from build123d import *

# Parameters (mm, degrees)
SKETCH_1_W      = 42
SKETCH_1_H      = 60
SKETCH_1_R      = 8
SKETCH_1_R_2    = 1.6
SKETCH_1_R_3    = 2.5
EXTRUDE_1_DEPTH = 2


with BuildPart() as part:
    # 草图1 → 凸台-拉伸1 (new body)
    with BuildSketch(Plane.XY):
        with Locations((0, -9)):
            Rectangle(SKETCH_1_W, SKETCH_1_H)
        Circle(SKETCH_1_R, mode=Mode.SUBTRACT)
        with Locations((-15.5, 15.5)):
            Circle(SKETCH_1_R_2, mode=Mode.SUBTRACT)
        with Locations((-15.5, -15.5)):
            Circle(SKETCH_1_R_2, mode=Mode.SUBTRACT)
        with Locations((-12.5, -31)):
            Circle(SKETCH_1_R_3, mode=Mode.SUBTRACT)
        with Locations(Location((15.5, 15.5, 0), (0, 0, 180))):
            Circle(SKETCH_1_R_2, mode=Mode.SUBTRACT)
        with Locations(Location((15.5, -15.5, 0), (0, 0, 180))):
            Circle(SKETCH_1_R_2, mode=Mode.SUBTRACT)
        with Locations(Location((12.5, -31, 0), (0, 0, 180))):
            Circle(SKETCH_1_R_3, mode=Mode.SUBTRACT)
    extrude(amount=EXTRUDE_1_DEPTH)


solid = part.part
Source: CAD feature listing. Evaluate the final solid. Frame: model axes, mm. Round coordinates to 2 decimals unless told otherwise and drop trailing zeros. Order: outer loops, then holes, each group sorted by start corner. A loop starts at its lowest first (then second) coordinate and runs counter-clockwise, first axis right, second up. Notation, with made-up numbers: (23.5, 64) - (73.5, 64) arc R27 ccw to (73.5, 82) - close; hole circle Ø7 at (34, 28). An arc over 180 degrees is marked (long way). Use a Markdown table: item, result. Add a question column.
1. Line query: probe 1 along Y at (x, z) = (-15.5, 0.45); probe 2 along Y at (x, z) = (-12.5, 0.95); probe 3 along Y at (x, z) = (-14.5, 1.5). Output: solid intervals per line, ascending.
2. Section query D-D (z = 1.15). Return the cut outline in (x, y).
3. Section query C-C (y = 15.5). Return the cut outline in (x, z).
4. Mould query, pull axis X, two halves, no side actions, for faces 1 (the cylindrical face through (16.68, -16.58, 0.99)), 2 (the flat face through (0, -39, 1)), 3 (the cylindrical face through (14, -33, 1)), 4 (the flat face through (-21, -9, 1)). Classes: +X half, -X half, draft (parallel to the pull), parting line (faces both ways), or undercut.
5. Section query B-B (x = -12.5). Return the cut outline in (y, z), then the cut area to 3 significant figures.
6. Section query A-A (y = 0). Return the cut outline in (x, z).
Derived:
| question | item | result |
|---|---|---|
| 1 | probe 1 | -39 to -17.1, -13.9 to 13.9, 17.1 to 21 |
| 1 | probe 2 | -39 to -33.5, -28.5 to 21 |
| 1 | probe 3 | -39 to -32.5, -29.5 to -16.75, -14.25 to 14.25, 16.75 to 21 |
| 2 | outline | (-21, -39) - (21, -39) - (21, 21) - (-21, 21) - close; hole circle Ø3.2 at (-15.5, -15.5); hole circle Ø3.2 at (-15.5, 15.5); hole circle Ø5 at (-12.5, -31); hole circle Ø16 at (0, 0); hole circle Ø5 at (12.5, -31); hole circle Ø3.2 at (15.5, -15.5); hole circle Ø3.2 at (15.5, 15.5) |
| 3 | outline | (-21, 0) - (-17.1, 0) - (-17.1, 2) - (-21, 2) - close; (-13.9, 0) - (13.9, 0) - (13.9, 2) - (-13.9, 2) - close; (17.1, 0) - (21, 0) - (21, 2) - (17.1, 2) - close |
| 4 | face 1 | undercut |
| 4 | face 2 | draft |
| 4 | face 3 | undercut |
| 4 | face 4 | -X half |
| 5 | outline | (-39, 0) - (-33.5, 0) - (-33.5, 2) - (-39, 2) - close; (-28.5, 0) - (21, 0) - (21, 2) - (-28.5, 2) - close |
| 5 | area | 110 mm2 |
| 6 | outline | (-21, 0) - (-8, 0) - (-8, 2) - (-21, 2) - close; (8, 0) - (21, 0) - (21, 2) - (8, 2) - close |
